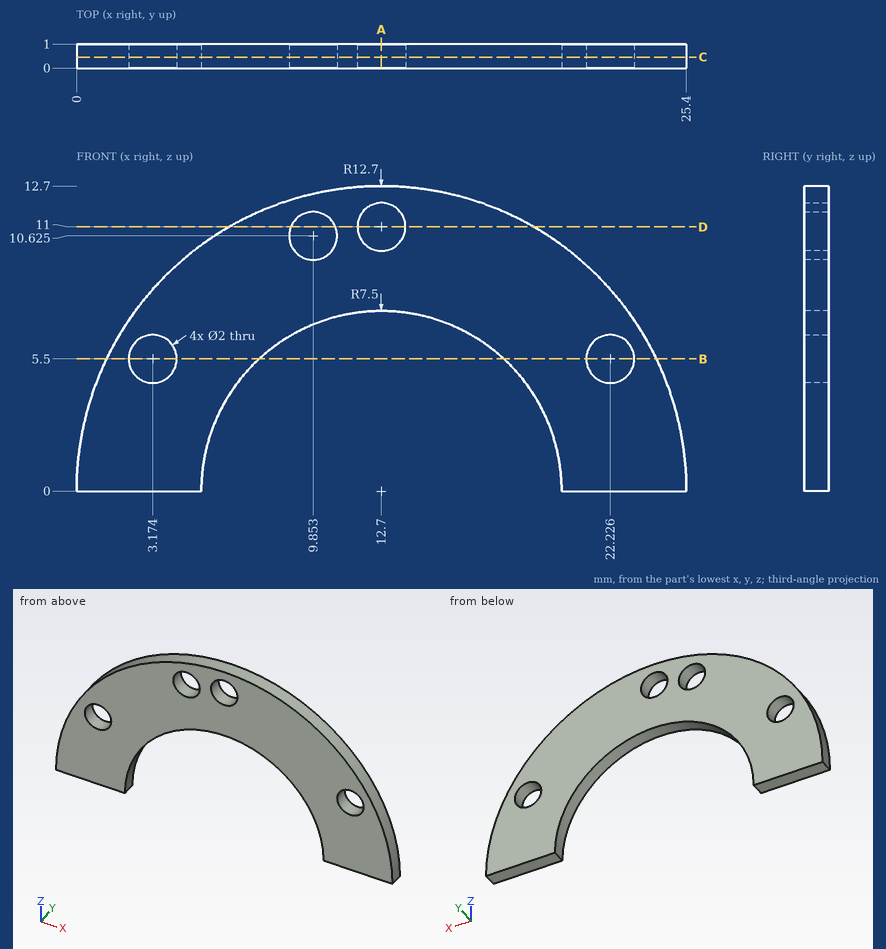
Answer from the drawing. Dimensions are ordinates in mm from the lowest x, y and z of the part. Coordinates: 2 decimals unless noted, no trailing zeros. Loops run counter-clockwise (first coordinate to the right, second up) from the corner with the lowest first, then second, coordinate; pieces in that order, holes last. Notation, with made-up numbers: (4.5, 38) - (25.5, 38) arc R23 cw to (25.5, 64) - close; hole circle Ø8 at (62, -34). An arc over 180 degrees is marked (long way). Answer in a Markdown table with one row per item.
1. Find section C-C, the plane y = 0.45. Write down the section's boundary in (x, z) (1 decimal), then the cut area to 3 significant figures.
Conclusion:
| item | result |
|---|---|
| outline | (0, 0) - (5.2, 0) arc R7.5 cw to (20.2, 0) - (25.4, 0) arc R12.7 ccw to start; hole circle Ø2 at (3.2, 5.5); hole circle Ø2 at (9.9, 10.6); hole circle Ø2 at (12.7, 11); hole circle Ø2 at (22.2, 5.5) |
| area | 152 mm² |
2. Find section D-D, the plane z = 11. Write down the section's boundary in (x, y).
Conclusion:
| item | result |
|---|---|
| outline | (6.35, 0) - (8.93, 0) - (8.93, 1) - (6.35, 1) - close; (10.78, 0) - (11.7, 0) - (11.7, 1) - (10.78, 1) - close; (13.7, 0) - (19.05, 0) - (19.05, 1) - (13.7, 1) - close |
3. Find section B-B, the plane z = 5.5. Write down the section's boundary in (x, y).
Conclusion:
| item | result |
|---|---|
| outline | (1.25, 0) - (2.17, 0) - (2.17, 1) - (1.25, 1) - close; (4.17, 0) - (7.6, 0) - (7.6, 1) - (4.17, 1) - close; (17.8, 0) - (21.23, 0) - (21.23, 1) - (17.8, 1) - close; (23.23, 0) - (24.15, 0) - (24.15, 1) - (23.23, 1) - close |
4. Straight lines are drawn through the part: line 1 (X direction, y = 0.65, z = 5.5) (1 decimal); line 2 (Z direction, x = 10.25, y = 0.85); line 3 (Z direction, x = 10.5, y = 0.4). For each, find the intervals that lie inside material, in ascending order.
Conclusion:
| item | result |
|---|---|
| line 1 | x = 1.3 to 2.2, 4.2 to 7.6, 17.8 to 21.2, 23.2 to 24.1 |
| line 2 | z = 7.09 to 9.71, 11.54 to 12.46 |
| line 3 | z = 7.17 to 9.86, 11.39 to 12.51 |
5. Find section A-A, the plane x = 12.7. Write down the section's boundary in (y, z).
Conclusion:
| item | result |
|---|---|
| outline | (0, 7.5) - (1, 7.5) - (1, 10) - (0, 10) - close; (0, 12) - (1, 12) - (1, 12.7) - (0, 12.7) - close |
6. Given pin 1 (1.8 mm diameter, centred on x = 9.85, z = 10.63, fed in from -Y), flat-ended and moving along its own axis, determine where the tip first touches the part or whether it passes through.
Conclusion:
| item | result |
|---|---|
| pin 1 | passes through |
